Here's the drawing with two shaded views (mm, measured from the low corner). I have some questions. Give positions to 0.01 mm unless a question says otherwise; leave off trailing zeros. Loops run counter-clockwise (first coordinate to the right, second up) from the corner with the lowest first, then second, coordinate; pieces in that order, holes last. Notation, with made-up numbers: (8.25, 71) - (46.25, 71) arc R24 ccw to (46.25, 108) - close; hole circle Ø6 at (74.25, -21.5). An arc over 180 degrees is marked (long way). Use one line per item in the form item = value.
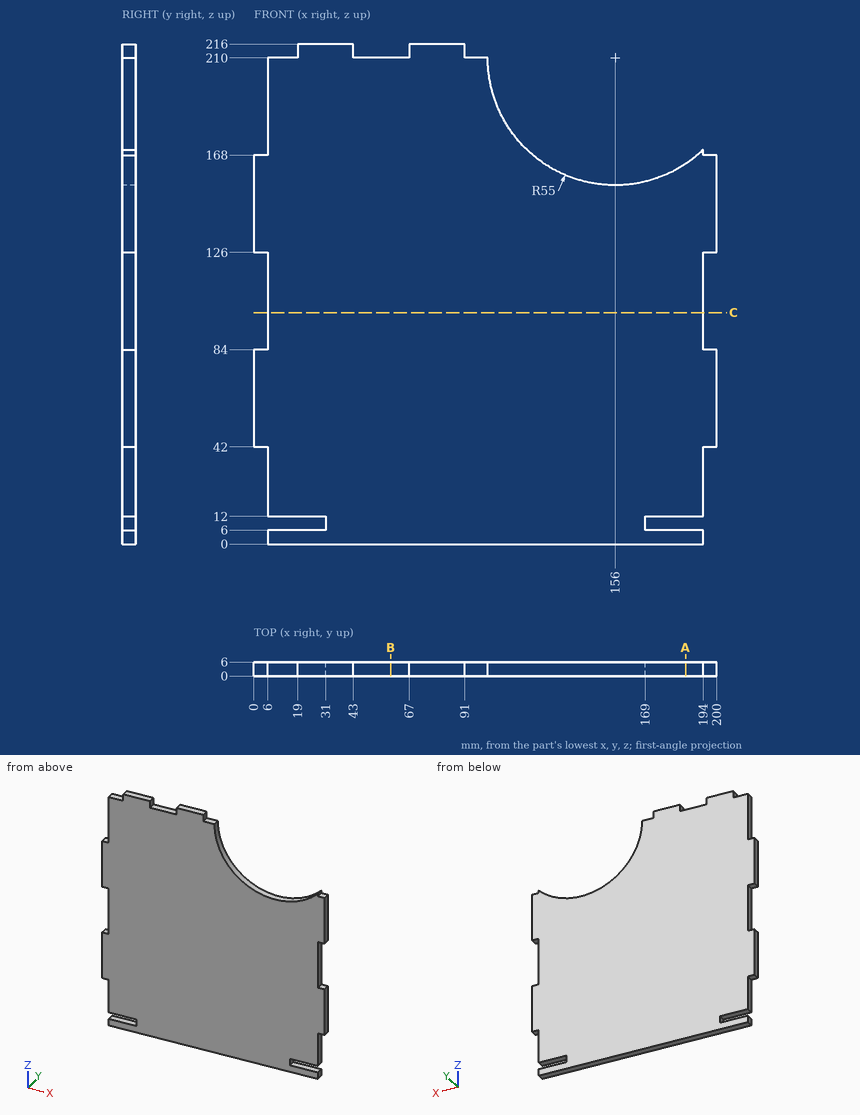
(1) If I drill on probe 1 along Z at (x, y) = (16, 3.1); probe 2 along Z at (x, y) = (176, 1.8); probe 3 along X at (y, z) = (3.5, 161), over which ranges is the centre line in solid material (lowest first)?
Geometry says:
probe_1 = 0 to 6, 12 to 210
probe_2 = 0 to 6, 12 to 158.77
probe_3 = 0 to 131.02, 180.98 to 200
(2) If we section it at A-A (x = 186.5): List the corners of the cut face in (y, z) for me, plus the area to 3 significant figures.
Geometry says:
outline = (0, 0) - (6, 0) - (6, 6) - (0, 6) - close; (0, 12) - (6, 12) - (6, 164.23) - (0, 164.23) - close
area = 949 mm²
(3) If we section it at B-B (x = 59): List the corners of the cut face in (y, z) for me.
Geometry says:
outline = (0, 0) - (6, 0) - (6, 210) - (0, 210) - close
(4) If we section it at C-C (z = 100): List the corners of the cut face in (x, y) for me, plus the area to 3 significant figures.
Geometry says:
outline = (6, 0) - (194, 0) - (194, 6) - (6, 6) - close
area = 1,130 mm²
(5) For P1, Ø3, axis at y = 2, z = 27, coming from the +X side; P2, Ø3, axis at y = 4.5, z = 33.5, coming from the -X side; P3, Ø1.8, axis at y = 2.5, z = 8.5, coming from the -X side, each with a flat end and sliding along its axis, tell me the tip position at first contact or that it passes through.
Geometry says:
P1 = 194
P2 = 6
P3 = 31
